Geometry check sheet. Reference: the model listing, model coordinates, mm. A direction names the side the tool comes from. Coordinates: 2 decimals unless noted, no trailing zeros. Order: outer loops, then holes, each group sorted by start corner. A loop starts at its lowest first (then second) coordinate and runs counter-clockwise, first axis right, second up.
```python
from build123d import *

# Parameters (mm, degrees)
SKETCH1_W           = 19.05
SKETCH1_H           = 30.48
BOSS_EXTRUDE1_DEPTH = 20.32
FILLET1_R           = 3.175
SKETCH2_R           = 6
BOSS_EXTRUDE2_DEPTH = 6.35
SKETCH3_W           = 12.7
SKETCH3_H           = 1.27
BOSS_EXTRUDE3_DEPTH = 7.62
SKETCH4_W           = 25.4
SKETCH4_H           = 43.18
BOSS_EXTRUDE4_DEPTH = 1.27
SKETCH5_R           = 3
BOSS_EXTRUDE5_DEPTH = 10


with BuildPart() as part:
    # Sketch1 → Boss-Extrude1 (new body)
    with BuildSketch(Plane(origin=(0, 0, 0), x_dir=(1, 0, 0), z_dir=(0, 1, 0))):
        Rectangle(SKETCH1_W, SKETCH1_H)
    extrude(amount=BOSS_EXTRUDE1_DEPTH)

    # Fillet1
    fillet1_edges = [part.edges().sort_by_distance(p)[0] for p in [
        (9.525, 10.16, 15.24),
        (-9.525, 10.16, 15.24),
        (-9.525, 10.16, -15.24),
        (9.525, 10.16, -15.24),
    ]]
    fillet(fillet1_edges, radius=FILLET1_R)

    # Sketch2 → Boss-Extrude2 (add)
    with BuildSketch(Plane(origin=(0, 20.32, 0), x_dir=(1, 0, 0), z_dir=(0, 1, 0))):
        Circle(SKETCH2_R)
    extrude(amount=BOSS_EXTRUDE2_DEPTH)

    # Sketch3 → Boss-Extrude3 (add)
    with BuildSketch(Plane.XZ):
        with Locations((0, 13.335)):
            Rectangle(SKETCH3_W, SKETCH3_H)
        with Locations((0, -13.335)):
            Rectangle(SKETCH3_W, SKETCH3_H)
    extrude(amount=BOSS_EXTRUDE3_DEPTH)

    # Sketch4 → Boss-Extrude4 (add)
    with BuildSketch(Plane(origin=(0, 26.67, 0), x_dir=(1, 0, 0), z_dir=(0, 1, 0))):
        with Locations((0, 6.35)):
            Rectangle(SKETCH4_W, SKETCH4_H)
    extrude(amount=BOSS_EXTRUDE4_DEPTH)

    # Sketch5 → Boss-Extrude5 (add)
    with BuildSketch(Plane(origin=(0, 27.94, 0), x_dir=(1, 0, 0), z_dir=(0, 1, 0))):
        Circle(SKETCH5_R)
    extrude(amount=BOSS_EXTRUDE5_DEPTH)


solid = part.part
```
Item 1: Release check for a two-part mould opening along Y. For faces 1 (the face through (-6, 23, 0)), 2 (the face through (0, -7.62, -13)), 3 (the face through (-6.5, 20.32, -0.2)), 4 (the face through (0, 10, 15.24)) record: pulls with the +Y half, pulls with the -Y half, needs draft (parallel to the pull), parting line crosses it, or undercut.
Item 2: Sectioned sample at D-D (y = 11.5). Record the cut outline in (x, z) (3 decimals).
Item 3: Sectioned sample at A-A (x = 0). Record the cut outline in (y, z), and give its area (3 significant figures).
Item 4: Thickness scan on line 1 along Z through (x, y) = (5.75, -1); line 2 along Y through (x, z) = (-5.75, -9); line 3 along Y through (x, z) = (11.25, -14). Record the ranges inside material, lowest first.
Item 5: Sectioned sample at C-C (z = 0). Record the cut outline in (x, y) (3 decimals).
Item 6: Tool access check on faces 5 (the face through (8.57, 10.302, 14.335)), 6 (the face through (-3, 33, 0)), 7 (the face through (0, -4, -13.97)), 8 (the face through (-6.35, -4, 13)), 9 (the face through (0, -4, 13.97)). Record the directions out of +Z, -Z, +X, -X, +Y, -Y that give a thin tool (end or side, any length) a straight path to the whole face; none if there is none.
Item 7: Sectioned sample at B-B (y = -3.5). Record the cut outline in (x, z), and give its area (3 significant figures).
Item 8: Depth check by flat-ended pin: P1, Ø1, axis at x = 8.5, z = -12.5, coming from the +Y side; P2, Ø1.5, axis at x = -8, z = -6, coming from the -Y side; P3, Ø0.6, axis at y = -5.5, z = -13, coming from the -X side; P4, Ø8, axis at y = 20, z = -22.5, coming from the +X side. Enter the tip coordinate at first touch or a pass-through.
Geometry check:
1. face 1: undercut
1. face 2: pulls with the -Y half
1. face 3: undercut
1. face 4: needs draft
2. outline: (-9.525, -12.065) arc R3.175 ccw to (-6.35, -15.24) - (6.35, -15.24) arc R3.175 ccw to (9.525, -12.065) - (9.525, 12.065) arc R3.175 ccw to (6.35, 15.24) - (-6.35, 15.24) arc R3.175 ccw to (-9.525, 12.065) - close
3. outline: (-7.62, -13.97) - (0, -13.97) - (0, -15.24) - (20.32, -15.24) - (20.32, -6) - (26.67, -6) - (26.67, -27.94) - (27.94, -27.94) - (27.94, -3) - (37.94, -3) - (37.94, 3) - (27.94, 3) - (27.94, 15.24) - (26.67, 15.24) - (26.67, 6) - (20.32, 6) - (20.32, 15.24) - (0, 15.24) - (0, 13.97) - (-7.62, 13.97) - (-7.62, 12.7) - (0, 12.7) - (0, -12.7) - (-7.62, -12.7) - close
3. area: 830 mm2
4. line 1: z = -13.97 to -12.7, 12.7 to 13.97
4. line 2: y = 0 to 20.32, 26.67 to 27.94
4. line 3: y = 26.67 to 27.94
5. outline: (-12.7, 26.67) - (-6, 26.67) - (-6, 20.32) - (-9.525, 20.32) - (-9.525, 0) - (9.525, 0) - (9.525, 20.32) - (6, 20.32) - (6, 26.67) - (12.7, 26.67) - (12.7, 27.94) - (3, 27.94) - (3, 37.94) - (-3, 37.94) - (-3, 27.94) - (-12.7, 27.94) - close
6. face 5: +Z, +X, -Y
6. face 6: +Y
6. face 7: -Z, +X, -X, -Y
6. face 8: +Z, -Z, -X, -Y
6. face 9: +Z, +X, -X, -Y
7. outline: (-6.35, -13.97) - (6.35, -13.97) - (6.35, -12.7) - (-6.35, -12.7) - close; (-6.35, 12.7) - (6.35, 12.7) - (6.35, 13.97) - (-6.35, 13.97) - close
7. area: 32.3 mm2
8. P1: stops at y = 27.94
8. P2: stops at y = 0
8. P3: stops at x = -6.35
8. P4: passes through
